Here's how the part is built. I have some questions about the finished solid (model axes, mm). Give positions to 0.01 mm unless a question says otherwise; leave off trailing zeros. Write each loop counter-clockwise with the first axis right and the second up, starting at its lowest first coordinate (ties: lowest second). Pieces come first, ordered by that corner, then holes. Notation, with made-up numbers: (54.25, 33) - (89.25, 33) arc R21 ccw to (89.25, 64) - close; hole circle Ø10 at (68, 43). An arc over 180 degrees is marked (long way). Write each question's results on one line, items separated by ' | '. Start each with the question number.
Item 1: Suppose I cut it at D-D on y = -0.75. List the corners of the cut face in (x, z) for me.
Item 2: Suppose I cut it at C-C on y = -5. List the corners of the cut face in (x, z) for me.
Item 3: We'd pull the mould along X, two halves only. Please class faces 1 (the cylindrical face through (-13.887, -2.169, -10.648)), 2 (the cylindrical face through (0.26, -3.11, 8.33)), 3 (the flat face through (5, -6.3, -5)): +X half, -X half, draft (parallel to the pull), parting line (faces both ways), or undercut.
Item 4: Suppose I cut it at A-A on x = 0. List the corners of the cut face in (y, z) for me.
Item 5: Please list where these lines run through material, in increasing order: line 1 along Z through (x, y) = (0, -3); line 2 along Z through (x, y) = (-1, -3.5); line 3 along X through (y, z) = (-4, -1.5).
Item 6: Will these pins go through, and if not, where does the flat tip stop? P1, Ø3, axis at x = 3.5, y = -3.5, coming from the +Z side; P2, Ø1.9, axis at x = 0, z = -9.5, coming from the -Y side.
Item 7: Suppose I cut it at B-B on z = 0. List the corners of the cut face in (x, y) for me.
```python
from build123d import *

# Parameters (mm, degrees)
F0_R     = 17.5
F0_R_2   = 6
F1_DEPTH = 6.3
F2_SIZE2 = 1.9
F2_SIZE  = 5.7
F4_D     = 2.4


with BuildPart() as f1:
    # F0 (on Front) → F1 (new body)
    with BuildSketch(Plane.XZ):
        Circle(F0_R)
        Circle(F0_R_2, mode=Mode.SUBTRACT)
    extrude(amount=F1_DEPTH)

    # F2
    f2_edges = [f1.edges().sort_by_distance(p)[0] for p in [
        (-17.5, -6.3, 0),
    ]]
    f2_side = f1.faces().sort_by_distance((-17.005025, -6.3, 0))[0]
    chamfer(f2_edges, length=F2_SIZE, length2=F2_SIZE2, reference=f2_side)

    # F4 (through all)
    with Locations(Plane.XZ.offset(6.3)):
        with Locations((0, 9.5), (-8, 0), (0, -9.5), (8, 0)):
            Hole(F4_D / 2)


solid = f1.part
```
Checked values:
1) outline: circle Ø35 at (0, 0); hole circle Ø2.4 at (-8, 0); hole circle Ø12 at (0, 0); hole circle Ø2.4 at (0, -9.5); hole circle Ø2.4 at (0, 9.5); hole circle Ø2.4 at (8, 0)
2) outline: circle Ø31.4 at (0, 0); hole circle Ø2.4 at (-8, 0); hole circle Ø12 at (0, 0); hole circle Ø2.4 at (0, -9.5); hole circle Ø2.4 at (0, 9.5); hole circle Ø2.4 at (8, 0)
3) face 1: parting line | face 2: undercut | face 3: draft
4) outline: (-6.3, -11.8) - (-4.4, -17.5) - (0, -17.5) - (0, -10.7) - (-6.3, -10.7) - close; (-6.3, -8.3) - (0, -8.3) - (0, -6) - (-6.3, -6) - close; (-6.3, 6) - (0, 6) - (0, 8.3) - (-6.3, 8.3) - close; (-6.3, 10.7) - (0, 10.7) - (0, 17.5) - (-4.4, 17.5) - (-6.3, 11.8) - close
5) line 1: z = -17.5 to -10.7, -8.3 to -6, 6 to 8.3, 10.7 to 17.5 | line 2: z = -17.47 to -10.16, -8.84 to -5.92, 5.92 to 8.84, 10.16 to 17.47 | line 3: x = -17.44 to -5.81, 5.81 to 17.44
6) P1: stops at z = 17.39 | P2: passes through
7) outline: (-17.5, -4.4) - (-11.8, -6.3) - (-9.2, -6.3) - (-9.2, 0) - (-17.5, 0) - close; (-6.8, -6.3) - (-6, -6.3) - (-6, 0) - (-6.8, 0) - close; (6, -6.3) - (6.8, -6.3) - (6.8, 0) - (6, 0) - close; (9.2, -6.3) - (11.8, -6.3) - (17.5, -4.4) - (17.5, 0) - (9.2, 0) - close
